Answer from the drawing. Dimensions are ordinates in mm from the lowest x, y and z of the part. A direction names the side the tool comes from. Round coordinates to 2 decimals unless told otherwise and drop trailing zeros. Loops run counter-clockwise (first coordinate to the right, second up) from the corner with the lowest first, then second, coordinate; pieces in that order, holes last. Notation, with made-up numbers: M 61.25,58 L 86.25,58 A15 cw 86.25,64 Z; hole C -17,-2.5 d11. An arc over 180 degrees is marked long. One line per item, written item: value.
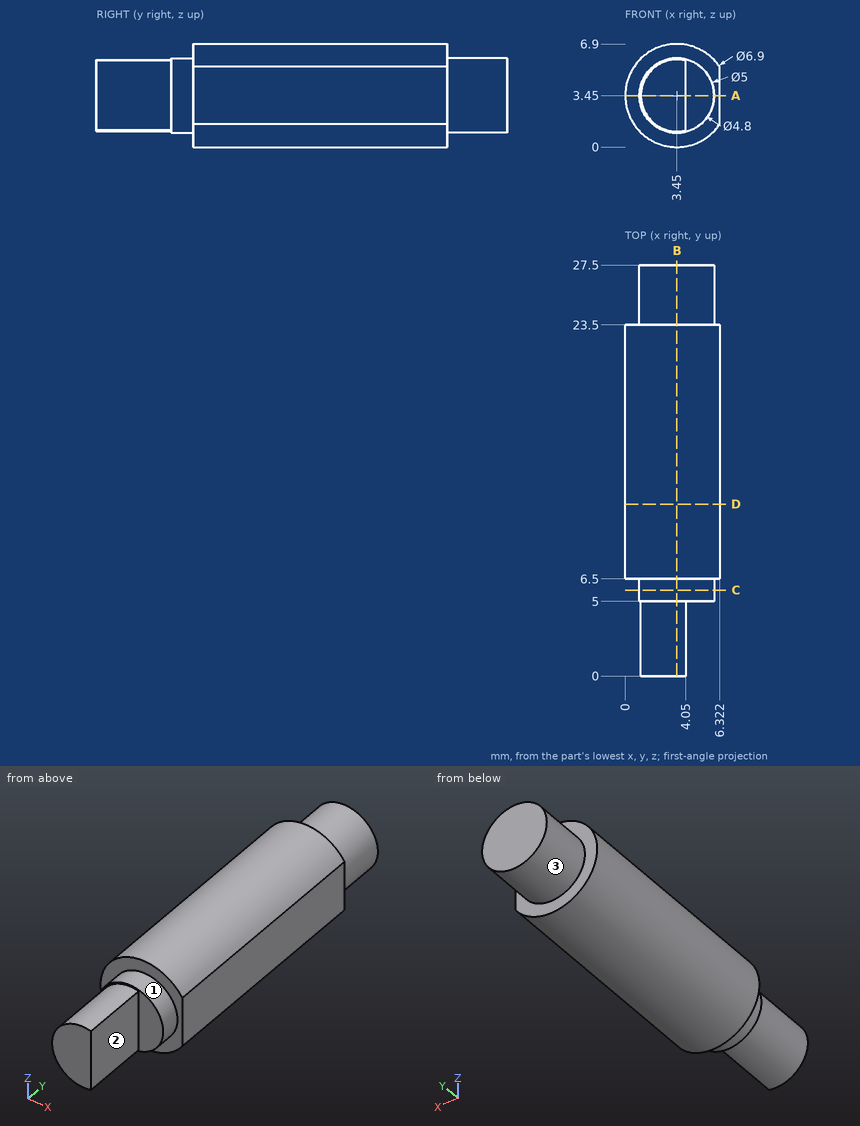
1) For the marked faces 1, 2 and 3, determine the directions among +Z, -Z, +X, -X, +Y, -Y from which every point of the face is accessible in a straight line to the end or side of a thin tool.
Check values:
face 1: -Y
face 2: +Z, -Z, +X, -Y
face 3: +Y
2) Find section B-B (x = 3.45). Give the vertices of the cut face in (y, z).
Check values:
outline: M 0,1.05 L 5,1.05 L 5,0.95 L 6.5,0.95 L 6.5,0 L 23.5,0 L 23.5,0.95 L 27.5,0.95 L 27.5,5.95 L 23.5,5.95 L 23.5,6.9 L 6.5,6.9 L 6.5,5.95 L 5,5.95 L 5,5.85 L 0,5.85 Z
3) Find the intervals of material crossed by probe 1 along Y at (x, z) = (2, 1); probe 2 along Y at (x, z) = (4.5, 5); probe 3 along Z at (x, y) = (2.25, 18.5) (1 decimal), in increasing order. Write a range as from..to.
Check values:
probe 1: 6.5..23.5
probe 2: 5..27.5
probe 3: 0.2..6.7
4) Each of these flat-tipped pins is pushed along its axis until it touches: pin 1 (3 mm diameter, centred on y = 21, z = 1.5, fed in from -X); pin 2 (1.4 mm diameter, centred on y = 2, z = 2.5, fed in from +X); pin 3 (1.5 mm diameter, centred on x = 2.5, z = 4, fed in from -Y). Where does it stop, or does it pass through?
Check values:
pin 1: x = 0.03
pin 2: x = 4.05
pin 3: y = 0
5) Find section D-D (y = 11.5). Give the vertices of the cut face in (x, z).
Check values:
outline: M 6.32,1.54 L 6.32,5.36 A3.45 ccw long Z
6) Find section C-C (y = 5.75). Give the vertices of the cut face in (x, z), then the cut area to 3 significant figures.
Check values:
outline: C 3.45,3.45 d5
area: 19.6 mm2
7) Find section A-A (z = 3.45). Give the vertices of the cut face in (x, y).
Check values:
outline: M 0,6.5 L 0.95,6.5 L 0.95,5 L 1.05,5 L 1.05,0 L 4.05,0 L 4.05,5 L 5.95,5 L 5.95,6.5 L 6.32,6.5 L 6.32,23.5 L 5.95,23.5 L 5.95,27.5 L 0.95,27.5 L 0.95,23.5 L 0,23.5 Z
